Check sheet for the modelled part. Datum: model origin and axes. Units: mm. Face numbers are marked on the shaded views. A direction names the side the tool comes from. Give positions to 0.01 mm unless a question says otherwise; leave off trailing zeros. Loops run counter-clockwise (first coordinate to the right, second up) from the corner with the lowest first, then second, coordinate; pieces in that order, holes last. Notation, with made-up numbers: (75, 60) - (102, 60) arc R25 ccw to (102, 99) - close; hole circle Ø10 at (39.5, 72.5). An arc over 180 degrees is marked (long way). Answer in a Markdown table with one row per item. Add a question column.
(1) Sectioned sample at D-D on z = 2.25. Enter the section's corners in (x, y).
(2) Sectioned sample at A-A on z = -0.25. Enter the section's corners in (x, y).
(3) Thickness scan on L1, parallel to Y at x = -3.95, z = 1; L2, parallel to Y at x = -4.3, z = 2.15; L3, parallel to X at y = 4.75, z = -0.5. Record the ranges inside material, lowest first.
(4) Go/stop test with flat-tipped pins: P1, Ø0.9, axis at x = -5, z = -0.5, coming from the -Y side; P2, Ø0.9, axis at y = 3.5, z = -0.5, coming from the +X side; P3, Ø0.6, axis at y = 3.5, z = -0.5, coming from the -X side. Record where each tip stops, or that it passes through.
(5) Set-up check for the marked faces 1, 2 and 3: record each of +Z, -Z, +X, -X, +Y, -Y from which the full face is reachable in a straight line by a thin tool's end or side.
(6) Sectioned sample at B-B on y = 4.5. Enter the section's corners in (x, z).
(7) Sectioned sample at C-C on x = -2.85. Enter the section's corners in (y, z), then the cut area to 3 significant figures.
(8) Draft check along Y on the marked faces 4, 5 and 6. Enter one of: released by +Y, released by -Y, zero draft, split by the parting line, or undercut.
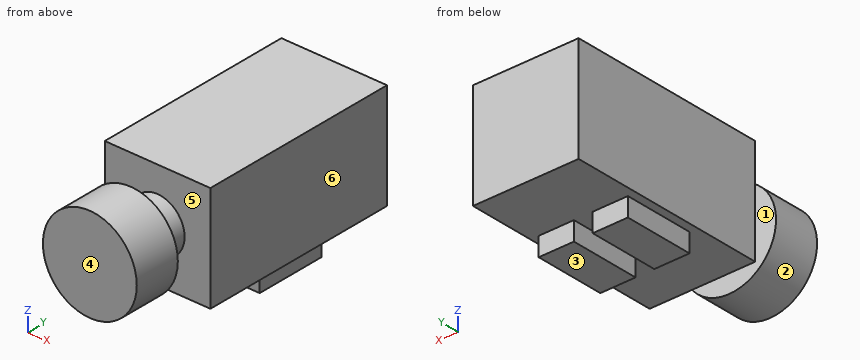
Autodesk Inventor part; units mm, degrees
ref_plane "YZ Plane" through (0, 0, 0) normal (1, 0, 0) x (0, 1, 0)
ref_plane "XZ Plane" through (0, 0, 0) normal (0, 1, 0) x (-1, 0, 0)
ref_plane "XY Plane" through (0, 0, 0) normal (0, 0, 1) x (1, 0, 0)
sketch "草图1" plane through (0, 0, 0) normal (0, 0, 1) x (1, 0, 0)
  line L0 (-6.0016, 8.0804) -> (-1.5016, 8.0804)
  line L1 (-1.5016, 8.0804) -> (-1.5016, -0.5196)
  line L2 (-1.5016, -0.5196) -> (-6.0016, -0.5196)
  line L3 (-6.0016, -0.5196) -> (-6.0016, 8.0804)
  line L4 (-3.7516, 8.0804) -> (-3.7516, -0.5196)
  line L5 (-3.3516, 5.2804) -> (-1.8516, 5.2804)
  line L6 (-1.8516, 5.2804) -> (-1.8516, 2.2804)
  line L7 (-1.8516, 2.2804) -> (-3.3516, 2.2804)
  line L8 (-3.3516, 2.2804) -> (-3.3516, 5.2804)
  line L9 (-4.1516, 5.2804) -> (-5.6516, 5.2804)
  line L10 (-5.6516, 5.2804) -> (-5.6516, 2.2804)
  line L11 (-5.6516, 2.2804) -> (-4.1516, 2.2804)
  line L12 (-4.1516, 2.2804) -> (-4.1516, 5.2804)
  point P0 (0, 0)
  dimension "d0" = 4.5
  dimension "d1" = 8.6
  dimension "d5" = 1.5
  dimension "d6" = 3
  dimension "d7" = 2.8
extrude "拉伸1" add sketch "草图1" along normal blind 4.5 contours L0 L4 L2 L3 | L0 L1 L2 L4 | L5 L6 L7 L8 | L12 L11 L10 L9
extrude "拉伸2" add sketch "草图1" against normal blind 0.8 contours L5 L6 L7 L8 | L12 L11 L10 L9
sketch "草图2" plane through (-6.0016, -0.5196, 0) normal (0, -1, 0) x (1, 0, 0)
  line L0 (0, 4.5) -> (4.5, 4.5)
  line L1 (2.25, 4.5) -> (2.25, 0)
  line L2 (4.5, 0) -> (0, 0)
  line L3 (4.5, 0) -> (4.5, 4.5)
  line L4 (4.5, 2.25) -> (0, 2.25)
  line L5 (0, 0) -> (0, 4.5)
  circle A0 centre (2.25, 2.25) radius 1.15
  point P0 (6.0016, 0)
  dimension "d10" = 2.3
extrude "拉伸3" add sketch "草图2" along normal blind 1 contours A0 L4 L1 | L1 L4 A0 | L4 L1 A0 | L4 A0 L1
sketch "草图3" plane through (-3.7516, -1.5196, 2.25) normal (0, -1, 0) x (1, 0, 0)
  circle A0 centre (0, 0) radius 0.5
  point P0 (3.7516, -2.25)
  dimension "d13" = 1
extrude "拉伸4" add sketch "草图3" along normal blind 2.3
sketch "草图4" plane through (-3.7516, -3.8196, 2.25) normal (0, -1, 0) x (1, 0, 0)
  circle A0 centre (0, 0) radius 2
  point P0 (3.7516, -2.25)
  dimension "d16" = 4
extrude "拉伸5" add sketch "草图4" against normal blind 2
properties part number "mortor"
Reply:
| question | item | result |
|---|---|---|
| 1 | outline | (-6, -0.52) - (-4.9, -0.52) - (-4.9, -1.52) - (-4.25, -1.52) - (-4.25, -1.82) - (-5.75, -1.82) - (-5.75, -3.82) - (-1.75, -3.82) - (-1.75, -1.82) - (-3.25, -1.82) - (-3.25, -1.52) - (-2.6, -1.52) - (-2.6, -0.52) - (-1.5, -0.52) - (-1.5, 8.08) - (-6, 8.08) - close |
| 2 | outline | (-5.65, 2.28) - (-4.15, 2.28) - (-4.15, 5.28) - (-5.65, 5.28) - close; (-3.35, 2.28) - (-1.85, 2.28) - (-1.85, 5.28) - (-3.35, 5.28) - close |
| 3 | L1 | -3.82 to -1.82, -0.52 to 8.08 |
| 3 | L2 | -3.82 to -1.82, -1.52 to 8.08 |
| 3 | L3 | -5.65 to -4.15, -3.35 to -1.85 |
| 4 | P1 | y = 2.28 |
| 4 | P2 | x = -1.85 |
| 4 | P3 | x = -5.65 |
| 5 | face 1 | none |
| 5 | face 2 | -Y |
| 5 | face 3 | -Z, +X, -X, +Y, -Y |
| 6 | outline | (-6, 0) - (-5.65, 0) - (-5.65, -0.8) - (-4.15, -0.8) - (-4.15, 0) - (-3.35, 0) - (-3.35, -0.8) - (-1.85, -0.8) - (-1.85, 0) - (-1.5, 0) - (-1.5, 4.5) - (-6, 4.5) - close |
| 7 | outline | (-3.82, 0.46) - (-1.82, 0.46) - (-1.82, 4.04) - (-3.82, 4.04) - close; (-1.52, 1.54) - (-0.52, 1.54) - (-0.52, 0) - (2.28, 0) - (2.28, -0.8) - (5.28, -0.8) - (5.28, 0) - (8.08, 0) - (8.08, 4.5) - (-0.52, 4.5) - (-0.52, 2.96) - (-1.52, 2.96) - close |
| 7 | area | 49.7 mm^2 |
| 8 | face 4 | released by -Y |
| 8 | face 5 | undercut |
| 8 | face 6 | zero draft |
